Solid Edge part; units mm, degrees
sketch "Sketch1" plane through (0, 0, 0) normal (0, 0, 1) x (1, 0, 0)
  circle A0 centre (0, 0) radius 17
  circle A1 centre (0, 0) radius 4
  circle A2 centre (8, 0) radius 1.15
  circle A3 centre (5.6569, 5.6569) radius 1.15
  circle A4 centre (0, 8) radius 1.15
  circle A5 centre (-5.6569, 5.6569) radius 1.15
  circle A6 centre (-8, 0) radius 1.15
  circle A7 centre (-5.6569, -5.6569) radius 1.15
  circle A8 centre (0, -8) radius 1.15
  circle A9 centre (5.6569, -5.6569) radius 1.15
  circle A10 centre (9.1924, 9.1924) radius 1.7
  circle A11 centre (-9.1924, 9.1924) radius 1.7
  circle A12 centre (-9.1924, -9.1924) radius 1.7
  circle A13 centre (9.1924, -9.1924) radius 1.7
extrude "Protrusion1" add sketch "Sketch1" along normal blind 4
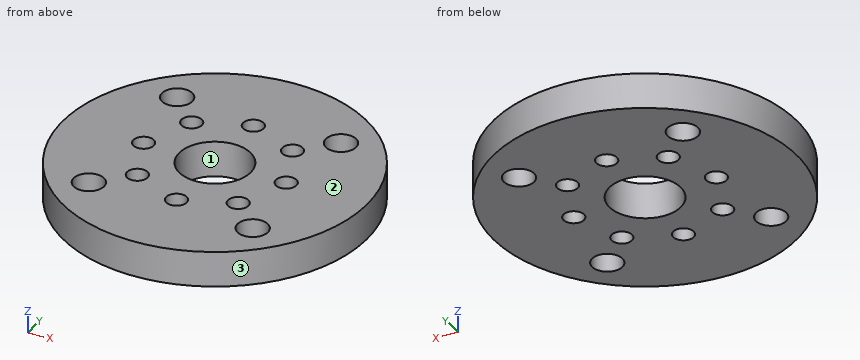
Input: part model. Units: mm. Frame: model coordinates. Face numbers are marked on the shaded views. Give positions to 0.01 mm unless a question says otherwise; leave off trailing zeros. Write each loop counter-clockwise with the first axis right and the second up, starting at its lowest first coordinate (ties: lowest second). Pieces come first, ordered by that corner, then holes. Notation, with made-up numbers: (-24, 42) -> (22, 42) arc R17 ccw to (22, 73) -> close; hole circle Ø10 at (-39.75, 58.5). An arc over 180 degrees is marked (long way). Use one line per item in the form item = value. Start each with the question number.
1) Ray query, probe 1 along Y at (x, z) = (0, 2.95); probe 2 along X at (y, z) = (10.5, 3.05); probe 3 along X at (y, z) = (6, 2.1). Return the intervals inside material, ascending. Write a range as from..to.
2) Section query A-A on y = 0. Return the cut outline in (x, z).
3) Pin query (flat end, axial travel): pin 1 (2 mm diameter, centred on y = 12, z = 2, fed in from -X); pin 2 (2.5 mm diameter, centred on x = 5.66, y = 5.66, fed in from -Z); pin 3 (1.4 mm diameter, centred on x = 0, y = -8, fed in from -Z); pin 4 (1.5 mm diameter, centred on y = 3, z = 1, fed in from -X). Return the tip coordinate at first contact, or that it passes through.
4) Section query D-D on z = 0.95. Count the separate pieces of the cut face and the enclosed holes in it, then the cut area to 3 significant figures.
5) Draft query along Y for the marked faces 1, 2 and 3. Return one class per face: pulls with the +Y half, pulls with the -Y half, needs draft (parallel to the pull), parting line crosses it, or undercut.
6) Section query C-C on y = 10. Return the cut outline in (x, z).
Outcome:
q1.probe_1 = -17..-9.15, -6.85..-4, 4..6.85, 9.15..17
q1.probe_2 = -13.37..-10.28, -8.11..8.11, 10.28..13.37
q1.probe_3 = -15.91..-6.75, -4.56..4.56, 6.75..15.91
q2.outline = (-17, 0) -> (-9.15, 0) -> (-9.15, 4) -> (-17, 4) -> close; (-6.85, 0) -> (-4, 0) -> (-4, 4) -> (-6.85, 4) -> close; (4, 0) -> (6.85, 0) -> (6.85, 4) -> (4, 4) -> close; (9.15, 0) -> (17, 0) -> (17, 4) -> (9.15, 4) -> close
q3.pin_1 = -12.96
q3.pin_2 = 0
q3.pin_3 = through
q3.pin_4 = -16.85
q4.separate_pieces = 1
q4.enclosed_holes = 13
q4.area = 788 mm^2
q5.face_1 = undercut
q5.face_2 = needs draft
q5.face_3 = parting line crosses it
q6.outline = (-13.75, 0) -> (-10.69, 0) -> (-10.69, 4) -> (-13.75, 4) -> close; (-7.7, 0) -> (7.7, 0) -> (7.7, 4) -> (-7.7, 4) -> close; (10.69, 0) -> (13.75, 0) -> (13.75, 4) -> (10.69, 4) -> close
